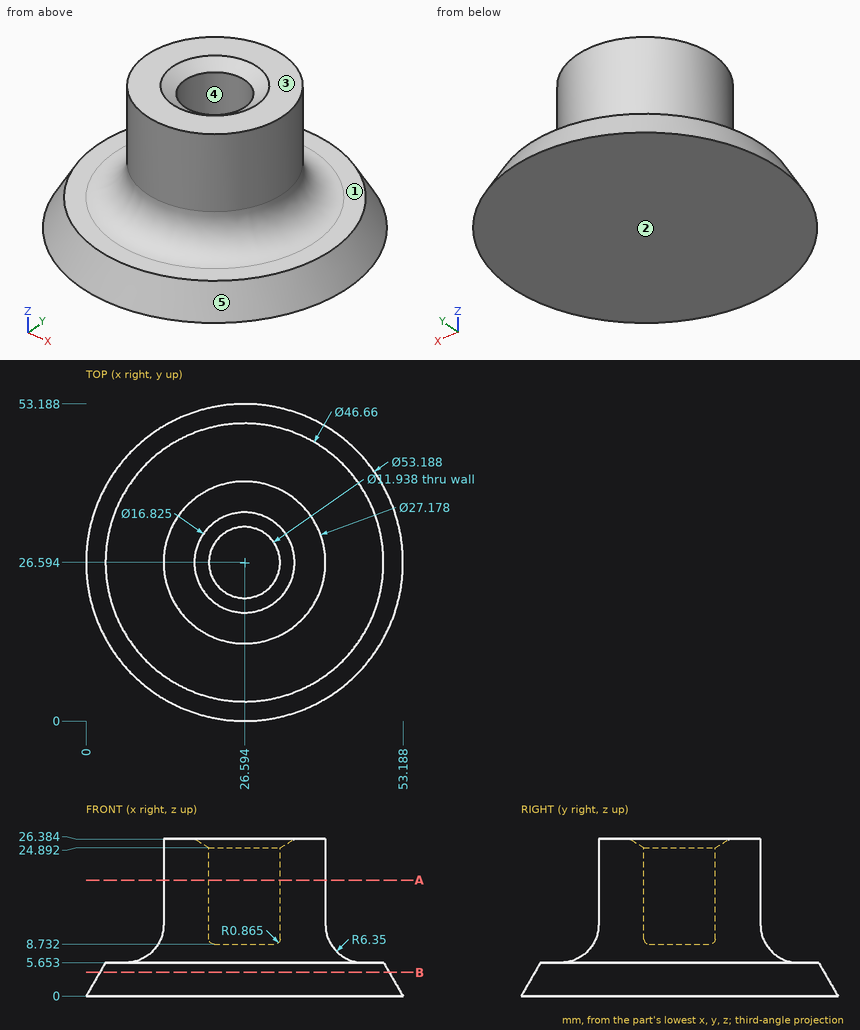
Geometry: see drawing. Coordinates: mm, zero at the bounding-box minimum. A direction names the side the tool comes from. Give positions to 0.01 mm unless a question says otherwise; leave off trailing zeros. Order: outer loops, then holes, each group sorted by start corner. A loop starts at its lowest first (then second) coordinate and runs counter-clockwise, first axis right, second up. Notation, with made-up numbers: (43, -22.5) -> (93, -22.5) arc R30 cw to (93, -0.5) -> close; hole circle Ø11 at (80, 82.25). An arc over 180 degrees is marked (long way). Write each question's results on one line, items separated by ' | '.
1) Set-up query: the marked faces 1 and 2. Return all of +Z, -Z, +X, -X, +Y, -Y with unobstructed straight access to the full face (end or side cutting, diameter ignored); none if empty.
Geometry says:
face 1: +Z | face 2: -Z, +X, -X, +Y, -Y
2) Cut plane B-B (z = 4). Output: boundary loops of the cut face in (x, y) (1 decimal), and give its area (3 significant figures).
Geometry says:
outline: circle Ø48.6 at (26.6, 26.6) | area: 1,850 mm²
3) Line query: line 1 along Z through (x, y) = (49, 27); line 2 along X through (y, z) = (14, 24) (1 decimal); line 3 along Y through (x, z) = (28.5, 18). Output: solid intervals per line, ascending.
Geometry says:
line 1: z = 0 to 5.65 | line 2: x = 21.5 to 31.7 | line 3: y = 13.14 to 20.94, 32.25 to 40.05
4) First-contact query: pin 1 Ø3 at (y, z) = (15.5, 21.5) entering from -X; pin 2 Ø10 at (x, y) = (11.5, 5.5) entering from -Z; pin 3 Ø6 at (x, z) = (31, 18.5) entering from +Y; pin 4 Ø8 at (x, z) = (25, 17.5) entering from +Y. Flat tips, straight axial feed; report the tip coordinate or a pass-through.
Geometry says:
pin 1: stops at x = 16.97 | pin 2: stops at z = 0 | pin 3: stops at y = 40.11 | pin 4: stops at y = 40.18
5) Cut plane A-A (z = 19.5). Output: boundary loops of the cut face in (x, y) (1 decimal).
Geometry says:
outline: circle Ø27.2 at (26.6, 26.6); hole circle Ø11.9 at (26.6, 26.6)
6) Draft query along Y for the marked faces 3, 4 and 5. Return one class per face: released by +Y, released by -Y, zero draft, split by the parting line, or undercut.
Geometry says:
face 3: zero draft | face 4: undercut | face 5: split by the parting line
